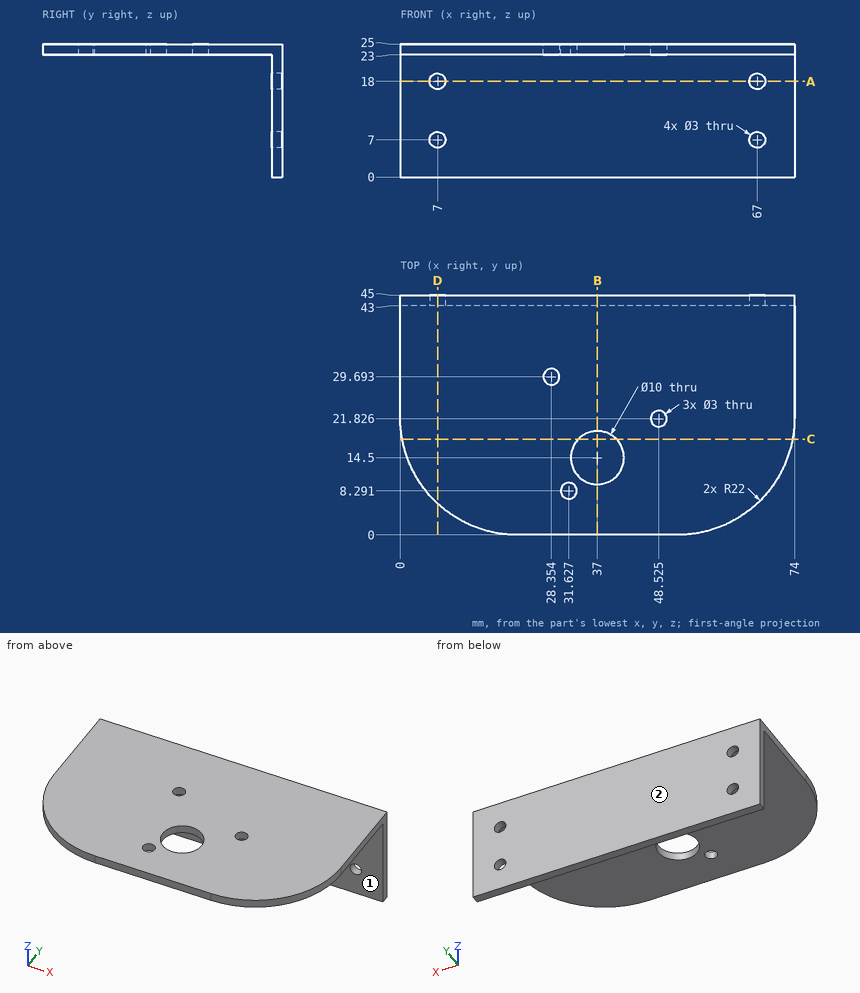
Design review of the part shown in the three views and the two pictorial views. Dimensions are in mm from the part's minimum x, y and z. A direction names the side the tool comes from. Give positions to 0.01 mm unless a question says otherwise; leave off trailing zeros. Loops run counter-clockwise (first coordinate to the right, second up) from the corner with the lowest first, then second, coordinate; pieces in that order, holes last. Notation, with made-up numbers: (-6, 28.5) - (50, 28.5) arc R21 ccw to (50, 52.5) - close; hole circle Ø2 at (-1.5, -30). An arc over 180 degrees is marked (long way). Answer as a JSON object with one key per item and string values.
Q1. Add section A-A on z = 18. State the section outline as (x, y) points.
Worked out:
{"outline": "(0, 43) - (5.5, 43) - (5.5, 45) - (0, 45) - close; (8.5, 43) - (65.5, 43) - (65.5, 45) - (8.5, 45) - close; (68.5, 43) - (74, 43) - (74, 45) - (68.5, 45) - close"}
Q2. For the marked faces 1 and 2, list the 3-axis set-ups (+Z, -Z, +X, -X, +Y, -Y) from which the entire face can be reached by the end or side of a thin tool; tool diameter is ignored.
Worked out:
{"face 1": "-Z, +X, -X, -Y", "face 2": "+Z, -Z, +X, -X, +Y"}
Q3. Add section D-D on x = 7. State the section outline as (y, z) points.
Worked out:
{"outline": "(5.91, 23) - (43, 23) - (43, 19.5) - (45, 19.5) - (45, 25) - (5.91, 25) - close; (43, 0) - (45, 0) - (45, 5.5) - (43, 5.5) - close; (43, 8.5) - (45, 8.5) - (45, 16.5) - (43, 16.5) - close"}
Q4. Add section C-C on y = 18. State the section outline as (x, z) points.
Worked out:
{"outline": "(0.37, 23) - (33.43, 23) - (33.43, 25) - (0.37, 25) - close; (40.57, 23) - (73.63, 23) - (73.63, 25) - (40.57, 25) - close"}
Q5. To check wall thickness, follow line 1 along X through (y, z) = (43.7, 7); line 2 along Z through (x, y) = (67, 43.4); line 3 along Y through (x, z) = (37, 23.8). State the ranges of each line that lie inside material, in increasing order.
Worked out:
{"line 1": "x = 0 to 5.5, 8.5 to 65.5, 68.5 to 74", "line 2": "z = 0 to 5.5, 8.5 to 16.5, 19.5 to 25", "line 3": "y = 0 to 9.5, 19.5 to 45"}
Q6. Insertion check: pin 1 (5 mm diameter, centred on x = 31.63, y = 8.29, fed in from +Z); pin 2 (3.5 mm diameter, centred on x = 7, z = 7, fed in from -Y); pin 3 (3.5 mm diameter, centred on x = 28.35, y = 29.69, fed in from -Z); pin 4 (8 mm diameter, centred on x = 37, y = 14.5, fed in from +Z). Each pin has a flat end and moves straight along its axis. Give the tip position at first contact, or say it passes through.
Worked out:
{"pin 1": "stops at z = 25", "pin 2": "stops at y = 43", "pin 3": "stops at z = 23", "pin 4": "passes through"}
Q7. Add section B-B on x = 37. State the section outline as (y, z) points, plus the area to 3 significant figures.
Worked out:
{"outline": "(0, 23) - (9.5, 23) - (9.5, 25) - (0, 25) - close; (19.5, 23) - (43, 23) - (43, 0) - (45, 0) - (45, 25) - (19.5, 25) - close", "area": "116 mm^2"}
